Read the model definition and answer for the solid it produces. Units are mm, in the model's axes. Face numbers are marked on the shaded views. A direction names the side the tool comes from. Coordinates: 2 decimals unless noted, no trailing zeros. Write each loop counter-clockwise with the first axis right and the second up, starting at its lowest first coordinate (ties: lowest second). Pieces come first, ordered by that corner, then holes.
from build123d import *

# Parameters (mm, degrees)
BOSS_EXTRUDE1_DEPTH = 5
SKETCH2_R           = 2.444777137
BOSS_EXTRUDE2_DEPTH = 3
SKETCH4_R           = 1.447783819
BOSS_EXTRUDE3_DEPTH = 48


with BuildPart() as part:
    # Sketch1 → Boss-Extrude1 (new body)
    with BuildSketch(Plane(origin=(0, 0, 0), x_dir=(1, 0, 0), z_dir=(0, 1, 0))):
        with BuildLine():
            Line((0, 16.15299729), (57.736574248, 16.15299729))
            ThreePointArc((57.736574248, 16.15299729), (72.459068519, -6.645862163), (45.621959745, -10.684354773))
            Line((45.621959745, -10.684354773), (12.114614503, -10.684354773))
            ThreePointArc((12.114614503, -10.684354773), (-14.722494271, -6.645862163), (0, 16.15299729))
        make_face()
    extrude(amount=BOSS_EXTRUDE1_DEPTH)

    # Sketch2 → Boss-Extrude2 (add)
    with BuildSketch(Plane(origin=(0, 0, 0), x_dir=(1, 0, 0), z_dir=(0, 1, 0))):
        with Locations(Location((-8.414564217, 7.18153284, 0), (0, 0, 270))):
            Circle(SKETCH2_R)
        with Locations(Location((-8.414564217, -7.18153284, 0), (0, 0, 270))):
            Circle(SKETCH2_R)
        with Locations(Location((8.414564217, 7.18153284, 0), (0, 0, 270))):
            Circle(SKETCH2_R)
        with Locations(Location((8.414564217, -7.18153284, 0), (0, 0, 270))):
            Circle(SKETCH2_R)
        with Locations(Location((66.151138464, 7.18153284, 0), (0, 0, 90))):
            Circle(SKETCH2_R)
        with Locations(Location((66.151138464, -7.18153284, 0), (0, 0, 90))):
            Circle(SKETCH2_R)
        with Locations(Location((49.322010031, -7.18153284, 0), (0, 0, 90))):
            Circle(SKETCH2_R)
        with Locations(Location((49.322010031, 7.18153284, 0), (0, 0, 90))):
            Circle(SKETCH2_R)
    extrude(amount=-BOSS_EXTRUDE2_DEPTH)

    # Sketch4 → Boss-Extrude3 (add)
    with BuildSketch(Plane(origin=(0, 0, -16.15299729), x_dir=(-1, 0, 0), z_dir=(0, 0, -1))):
        with Locations(Location((-28.970152838, 2.400681273, 0), (0, 0, 180))):
            Circle(SKETCH4_R)
    extrude(amount=BOSS_EXTRUDE3_DEPTH)


solid = part.part
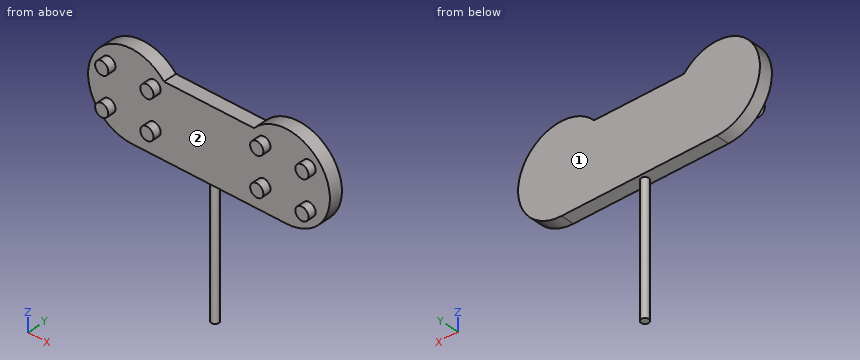
Item 1: The part is cut by section C-C (x = 35). Give the vertices of the cut face in (y, z).
Item 2: Given pin 1 (4 mm diameter, centred on y = 1, z = -9.5, fed in from +X); pin 2 (4 mm diameter, centred on x = 55.5, y = 1.5, fed in from -Z); pin 3 (1.5 mm diameter, centred on x = 26.5, y = 2, fed in from +Z); pin 4 (12 mm diameter, centred on x = 51, z = -11, fed in from -Y), each flat-ended and moving along its own axis, determine where each tip first touches the part or whether it passes through.
Item 3: The part is cut by section B-B (z = 7.5). Give the vertices of the cut face in (x, y), and give its area (3 significant figures).
Item 4: The part is cut by section A-A (x = -7). Give the vertices of the cut face in (y, z), and give its area (3 significant figures).
Item 5: For the marked faces 1 and 2, determine the directions among +Z, -Z, +X, -X, +Y, -Y from which every point of the face is accessible in a straight line to the end or side of a thin tool.
Item 6: Find the intervals of material crossed by probe 1 along Y at (x, z) = (-6.5, -3.5); probe 2 along Z at (x, y) = (29, 1); probe 3 along X at (y, z) = (-0.75, -9), in increasing order.
Item 7: The part is cut by section D-D (z = -46.5). Give the vertices of the cut face in (x, y), and give its area (3 significant figures).
Answer:
1. outline: (0, -16.15) - (5, -16.15) - (5, 10.68) - (0, 10.68) - close
2. pin 1: stops at x = 72.04
2. pin 2: stops at z = -16.15
2. pin 3: stops at z = 10.68
2. pin 4: stops at y = -3
3. outline: (-14.31, 0) - (-10.84, 0) - (-10.84, -3) - (-5.99, -3) - (-5.99, 0) - (5.99, 0) - (5.99, -3) - (10.84, -3) - (10.84, 0) - (46.9, 0) - (46.9, -3) - (51.75, -3) - (51.75, 0) - (63.73, 0) - (63.73, -3) - (68.58, -3) - (68.58, 0) - (72.04, 0) - (72.04, 5) - (-14.31, 5) - close
3. area: 490 mm2
4. outline: (-3, -9.18) - (0, -9.18) - (0, -14.56) - (5, -14.56) - (5, 14.56) - (0, 14.56) - (0, 9.18) - (-3, 9.18) - (-3, 5.19) - (0, 5.19) - (0, -5.19) - (-3, -5.19) - close
4. area: 170 mm2
5. face 1: +Z, -Z, +X, -X, +Y
5. face 2: -Y
6. probe 1: y = 0 to 5
6. probe 2: z = -64.15 to 10.68
6. probe 3: x = -10.05 to -6.78, 6.78 to 10.05, 47.69 to 50.96, 64.52 to 67.79
7. outline: circle Ø2.9 at (28.97, 2.4)
7. area: 6.59 mm2
